Part model, mm, in its own coordinate system. Give positions to 0.01 mm unless a question says otherwise; leave off trailing zeros. Loops run counter-clockwise (first coordinate to the right, second up) from the corner with the lowest first, then second, coordinate; pieces in that order, holes last. Notation, with made-up numbers: (-33, 80.5) -> (-16, 80.5) arc R10 ccw to (-16, 86.5) -> close; hole circle Ø9 at (3, -4.75). An arc over 180 degrees is marked (long way). Write item = value, one per line.
from build123d import *

# Parameters (mm, degrees)
BOSS_EXTRUDE1_DEPTH = 5
FILLET1_R           = 1


with BuildPart() as part:
    # Sketch1 → Boss-Extrude1 (new body)
    with BuildSketch(Plane(origin=(0, 0, 0), x_dir=(1, 0, 0), z_dir=(0, 1, 0))):
        Polygon((0, 0), (15, 25.980762114), (30, 0), align=None)
    extrude(amount=BOSS_EXTRUDE1_DEPTH)

    # Fillet1
    fillet1_edges = [part.edges().sort_by_distance(p)[0] for p in [
        (7.5, 5, -12.990381057),
        (7.5, 0, -12.990381057),
        (22.5, 0, -12.990381057),
        (15, 0, 0),
        (15, 5, 0),
        (0, 2.5, 0),
        (15, 2.5, -25.980762114),
        (30, 2.5, 0),
        (22.5, 5, -12.990381057),
    ]]
    fillet(fillet1_edges, radius=FILLET1_R)


solid = part.part
1) Drop flat-ended pins along their axis: P1, Ø1, axis at x = 4, z = -7.5, coming from the -Y side; P2, Ø3, axis at x = 5.5, y = 1, coming from the -Z side; P3, Ø2, axis at x = 25.5, y = 4.5, coming from the -Z side. Give the stop position or say it passes through.
Resolved:
P1 = 0.38
P2 = -12.12
P3 = -9.41
2) Drill centre lines: line 1 along Z through (x, y) = (23, 3.95); line 2 along Z through (x, y) = (21.25, 4.5); line 3 along X through (y, z) = (2.7, -17.75). Where is each one in solid material? Low to high. Write a range as [from, to].
Resolved:
line_1 = [-12.12, 0]
line_2 = [-14.89, -0.13]
line_3 = [10.25, 19.75]
3) Slice it at A-A, the plane y = 1.65. List the corners of the cut face in (x, z), and give its area (3 significant figures).
Resolved:
outline = (0.87, -1.5) -> (14.13, -24.48) arc R1 ccw to (15.87, -24.48) -> (29.13, -1.5) arc R1 ccw to (28.27, 0) -> (1.73, 0) arc R1 ccw to start
area = 388 mm²
